Source: CAD feature listing. Evaluate the final solid. Frame: model axes, mm. Face numbers are marked on the shaded views. Round coordinates to 2 decimals unless told otherwise and drop trailing zeros. Order: outer loops, then holes, each group sorted by start corner. A loop starts at its lowest first (then second) coordinate and runs counter-clockwise, first axis right, second up. Notation, with made-up numbers: M 3,38.25 L 36,38.25 A6 cw 36,46.25 Z; hole C 48,32.25 d1. An arc over 180 degrees is marked long. Answer as CSV lines item,"result". Start each with the question number.
Item 1: Section query B-B on y = -3.75. Return the cut outline in (x, z), plus the area to 3 significant figures.
Item 2: Line query: line 1 (Z direction, x = -40.5, y = -5.5); line 2 (Z direction, x = -44.45, y = -3); line 3 (X direction, y = -3, z = -33). Output: solid intervals per line, ascending. Write a range as [from, to].
Item 3: Section query D-D on x = -44.45. Return the cut outline in (y, z), plus the area to 3 significant figures.
Item 4: Pull-direction query (X, two-part tool) for the marked faces 1, 2 and 3; classes: +X half, -X half, draft (parallel to the pull), parting line (faces both ways), or undercut.
Item 5: Section query A-A on z = 0. Return the cut outline in (x, y), plus the area to 3 significant figures.
Item 6: First-contact query: P1, Ø8, axis at x = 44, z = -29.5, coming from the +Y side; P2, Ø6.5, axis at y = -5, z = -0.5, coming from the +X side; P3, Ø3, axis at x = 12, y = -8.5, coming from the +Z side. Flat tips, straight axial feed; report the tip coordinate or a pass-through.
Item 7: Section query C-C on z = -31. Return the cut outline in (x, y), plus the area to 3 significant figures.
from build123d import *

# Parameters (mm, degrees)
F0_R           = 63.5
F1_DEPTH       = 12.7
F3_DEPTH       = 25.4
F4_D           = 6.35
F4_CBORE_D     = 10.3124
F4_CBORE_DEPTH = 6.35


# Not quite as in the source:
# - a feature names something its author has since deleted; it is built from what else it names


with BuildPart() as f1:
    # F0 (on Front) → F1 (new body)
    with BuildSketch(Plane.XZ):
        Circle(F0_R)
    extrude(amount=F1_DEPTH)

    # F2 (on face) → F3 (cut)
    with BuildSketch(Plane.XZ.offset(12.7)):
        with BuildLine():
            Line((-7.93115, 63.0027527944), (-3.96875, 50.8))
            Line((-3.96875, 50.8), (-3.96875, -25.4))
            ThreePointArc((-3.96875, -25.4), (0, -29.36875), (3.96875, -25.4))
            Line((3.96875, -25.4), (3.96875, 50.8))
            Line((3.96875, 50.8), (7.93115, 63.0027527944))
            ThreePointArc((7.93115, 63.0027527944), (0, 63.5), (-7.93115, 63.0027527944))
        make_face()
    extrude(amount=-F3_DEPTH, mode=Mode.SUBTRACT)

    # F4 (through all)
    with Locations(Plane(origin=(0, 0, 0), x_dir=(1, 0, 0), z_dir=(0, 1, 0))):
        with Locations((44.45, -29.36875), (-44.45, -29.36875), (44.45, 29.36875), (-44.45, 29.36875)):
            CounterBoreHole(F4_D / 2, F4_CBORE_D / 2, F4_CBORE_DEPTH)


solid = f1.part
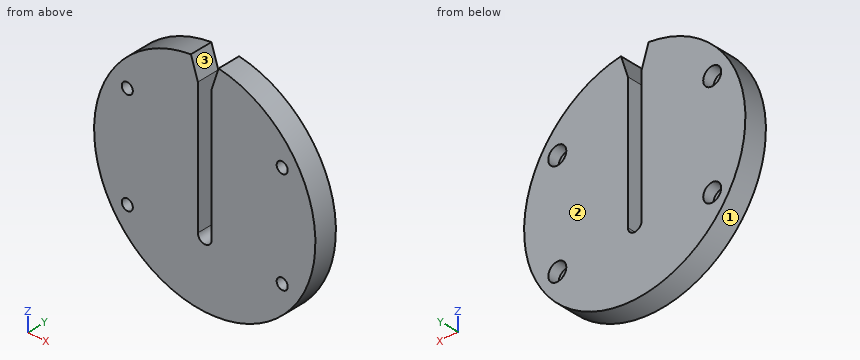
Results:
1,outline,"M -7.93,63 A63.5 ccw long 7.93,63 L 3.97,50.8 L 3.97,-25.4 A3.97 cw -3.97,-25.4 L -3.97,50.8 Z; hole C -44.45,-29.37 d10.31; hole C -44.45,29.37 d10.31; hole C 44.45,-29.37 d10.31; hole C 44.45,29.37 d10.31"
1,area,"11,600 mm^2"
2,line 1,"[-48.91, -32.68], [-26.05, 26.05], [32.68, 48.91]"
2,line 2,"[-45.35, -34.52], [-24.21, 24.21], [34.52, 45.35]"
2,line 3,"[-54.25, -48.11], [-40.79, 40.79], [48.11, 54.25]"
3,outline,"M -12.7,-45.35 L 0,-45.35 L 0,-34.52 L -6.35,-34.52 L -6.35,-32.54 L -12.7,-32.54 Z; M -12.7,-26.19 L -6.35,-26.19 L -6.35,-24.21 L 0,-24.21 L 0,24.21 L -6.35,24.21 L -6.35,26.19 L -12.7,26.19 Z; M -12.7,32.54 L -6.35,32.54 L -6.35,34.52 L 0,34.52 L 0,45.35 L -12.7,45.35 Z"
3,area,"940 mm^2"
4,face 1,"parting line"
4,face 2,"draft"
4,face 3,"undercut"
5,outline,"M -63.5,-12.7 L -3.97,-12.7 L -3.97,0 L -63.5,0 Z; M 3.97,-12.7 L 63.5,-12.7 L 63.5,0 L 3.97,0 Z"
5,area,"1,510 mm^2"
6,P1,"y = -6.35"
6,P2,"x = 63.5"
6,P3,"z = 62.63"
7,outline,"M -55.42,-12.7 L -47.17,-12.7 L -47.17,-6.35 L -49.34,-6.35 L -49.34,0 L -55.42,0 Z; M -41.73,-12.7 L 41.73,-12.7 L 41.73,-6.35 L 39.56,-6.35 L 39.56,0 L -39.56,0 L -39.56,-6.35 L -41.73,-6.35 Z; M 47.17,-12.7 L 55.42,-12.7 L 55.42,0 L 49.34,0 L 49.34,-6.35 L 47.17,-6.35 Z"
7,area,"1,210 mm^2"
